Geometry: final body of the model. Coordinates: model frame, mm. A direction names the side the tool comes from. Give positions to 0.01 mm unless a question says otherwise; leave off trailing zeros. Write each loop counter-clockwise with the first axis right and the second up, starting at its lowest first coordinate (ties: lowest second). Pieces come first, ordered by that corner, then holes.
Q1. Cut plane D-D on z = 16. Return the cut outline in (x, y) (3 decimals).
Q2. Reachability of faces 4 (the face through (-20.003, 7.013, 17.546)), 5 (the face through (-19.284, -19.4, 15.944)), 6 (the face through (0, -12.5, 3)) from +Z, -Z, +X, -X, +Y, -Y: full face, straight path, thin tool, end or side. Return the list, or none.
Q3. Line query: L1, parallel to X at y = -1.5, z = 13 (3 decimals); L2, parallel to Y at x = 13, z = 3.25; L3, parallel to Y at x = 0, z = 8.95. Output: solid intervals per line, ascending.
Q4. Cut plane C-C on x = 10. Return the cut outline in (y, z) (3 decimals).
Q5. Cut plane B-B on z = 3. Return the cut outline in (x, y), plus the area to 3 significant figures.
Q6. Draft query along Y for faces 1 (the face through (0, 22.5, 10)), 2 (the face through (3, 0, 6)), 3 (the face through (-22.5, 0, 10)). Return one class per face: pulls with the +Y half, pulls with the -Y half, needs draft (parallel to the pull), parting line crosses it, or undercut.
Q7. Cut plane A-A on y = -7.5. Return the cut outline in (x, z) (3 decimals), plus the area to 3 significant figures.
Q8. Pin query (flat end, axial travel): pin 1 (1.8 mm diameter, centred on x = 12.5, y = -12.5, fed in from -Z); pin 2 (3.5 mm diameter, centred on x = -12.5, y = -12.5, fed in from +Z); pin 3 (1.9 mm diameter, centred on x = 0, y = 0, fed in from -Z); pin 4 (6.5 mm diameter, centred on x = -17.575, y = 17.575, fed in from -Z). Return the tip coordinate at first contact, or that it passes through.
Autodesk Inventor part; units mm, degrees
ref_plane "YZ Plane" through (0, 0, 0) normal (1, 0, 0) x (0, 1, 0)
ref_plane "XZ Plane" through (0, 0, 0) normal (0, 1, 0) x (-1, 0, 0)
ref_plane "XY Plane" through (0, 0, 0) normal (0, 0, 1) x (1, 0, 0)
sketch "Sketch1" plane through (0, 0, 0) normal (0, 0, 1) x (1, 0, 0)
  line L0 (0, 31.5) -> (0, -31.5) construction
  line L1 (-31.5, 0) -> (31.5, 0) construction
  line L2 (-22.5, 22.5) -> (22.5, 22.5)
  line L3 (22.5, 22.5) -> (22.5, -22.5)
  line L4 (22.5, -22.5) -> (-22.5, -22.5)
  line L5 (-22.5, -22.5) -> (-22.5, 22.5)
  point P0 (0, 0)
  dimension "d0" = 45
  dimension "d1" = 45
extrude "Extrusion1" add sketch "Sketch1" along normal blind 20
sketch "Sketch4" plane through (0, 0, 20) normal (0, 0, 1) x (1, 0, 0)
  line L0 (-31.5, 0) -> (31.5, 0) construction
  line L1 (0, 31.5) -> (0, -31.5) construction
  line L2 (-17.575, 17.575) -> (17.575, 17.575) construction
  line L3 (17.575, 17.575) -> (17.575, -17.575) construction
  line L4 (17.575, -17.575) -> (-17.575, -17.575) construction
  line L5 (-17.575, -17.575) -> (-17.575, 17.575) construction
  point P0 (0, 0)
  dimension "d15" = 35.15
  dimension "d16" = 35.15
hole "Hole2" at (-17.575, 17.575, 20) at (17.575, 17.575, 20) at (17.575, -17.575, 20) at (-17.575, -17.575, 20) at (-17.575, 17.575, 20) at (17.575, 17.575, 20) direction (0, 0, -1) diameter 5 depth 8
sketch "Sketch5" plane through (0, 0, 20) normal (0, 0, 1) x (1, 0, 0)
  circle A0 centre (-17.575, 17.575) radius 2.5
  circle A1 centre (17.575, -17.575) radius 2.5
  line L0 (-17.575, 17.575) -> (17.575, 17.575)
  line L1 (17.575, 17.575) -> (17.575, -17.575)
  line L2 (17.575, -17.575) -> (-17.575, -17.575)
  line L3 (-17.575, -17.575) -> (-17.575, 17.575)
  point P0 (0, 0)
extrude "Extrusion3" cut sketch "Sketch5" against normal blind 8 contours L0 L1 A1 L2 L3 A0 | A0 L3 L0 | L1 L2 A1 picked at (-15.9292, 17.3896) picked at (17.028, -16.0118)
sketch "Sketch6" plane through (-22.5, -22.5, 0) normal (-1, 0, 0) x (0, 0, 1)
  line L0 (0, 45) -> (20, 45)
  line L1 (0, 0) -> (20, 0)
  line L2 (20, 7.425) -> (12, 7.425) construction
  line L3 (20, 37.575) -> (20, 7.425) construction
  line L4 (12, 37.575) -> (20, 37.575) construction
  line L5 (12, 7.425) -> (12, 37.575) construction
  line L6 (16, 37.575) -> (16, 7.425) construction
  point P0 (0, 22.5)
  point P1 (16, 30)
  point P2 (16, 15)
  dimension "d26" = 15
  dimension "d27" = 15
hole "Hole3" at (-22.5, 7.5, 16) at (-22.5, -7.5, 16) direction (1, 0, 0) diameter 3.242 end up to surface
sketch "Sketch8" plane through (0, 0, 0) normal (0, 0, -1) x (-1, 0, 0)
  line L0 (22.5, 22.5) -> (-22.5, 22.5) construction
  line L1 (-22.5, 22.5) -> (-22.5, -22.5) construction
  line L2 (-22.5, -22.5) -> (22.5, -22.5) construction
  line L3 (22.5, -22.5) -> (22.5, 22.5) construction
  line L4 (0, -38.5) -> (0, 38.5) construction
  line L5 (-38.5, 0) -> (38.5, 0) construction
  line L6 (-12.5, -12.5) -> (12.5, -12.5)
  line L7 (12.5, -12.5) -> (12.5, 12.5)
  line L8 (12.5, 12.5) -> (-12.5, 12.5)
  line L9 (-12.5, 12.5) -> (-12.5, -12.5)
  point P0 (0, 0)
  dimension "d44" = 25
  dimension "d45" = 25
extrude "Extrusion4" cut sketch "Sketch8" against normal blind 6
sketch "Sketch9" plane through (0, 0, 0) normal (0, 0, -1) x (-1, 0, 0)
  line L0 (12.5, 12.5) -> (12.5, -12.5) construction
  line L1 (12.5, -12.5) -> (-12.5, -12.5) construction
  line L2 (-12.5, -12.5) -> (-12.5, 12.5) construction
  line L3 (-12.5, 12.5) -> (12.5, 12.5) construction
  line L4 (22.5, 22.5) -> (-22.5, 22.5) construction
  line L5 (-22.5, 22.5) -> (-22.5, -22.5) construction
  line L6 (-22.5, -22.5) -> (22.5, -22.5) construction
  line L7 (22.5, -22.5) -> (22.5, 22.5) construction
  line L8 (12.5, -12.5) -> (-12.5, -12.5) construction
  point P0 (0, 0)
hole "Hole5" at (-12.5, 12.5, 0) at (-12.5, -12.5, 0) at (12.5, -12.5, 0) at (12.5, 12.5, 0) direction (0, 0, 1) diameter 3 depth 6
sketch "Sketch10" plane through (0, 0, 6) normal (0, 0, -1) x (-1, 0, 0)
  point P0 (0, 0)
  point P1 (0, 0)
hole "Hole6" at (0, 0, 6) direction (0, 0, 1) diameter 3.242 depth 4 tip angle 118
properties part number "Large-cuvette-mount-40mm-V3" material "PC/ABS Plastic"
Data:
1. outline: (-22.5, -22.5) - (22.5, -22.5) - (22.5, 22.5) - (-22.5, 22.5) - (-22.5, 9.121) - (-17.575, 9.121) - (-17.575, 15.075) arc R2.5 cw (long way) to (-15.075, 17.575) - (15.075, 17.575) arc R2.5 cw (long way) to (17.575, 15.075) - (17.575, -15.075) arc R2.5 cw (long way) to (15.075, -17.575) - (-15.075, -17.575) arc R2.5 cw (long way) to (-17.575, -15.075) - (-17.575, -9.121) - (-22.5, -9.121) - close; (-22.5, -5.879) - (-17.575, -5.879) - (-17.575, 5.879) - (-22.5, 5.879) - close
2. face 4: -X
2. face 5: +Z
2. face 6: -Z
3. L1: x = -22.5 to -17.575, 17.575 to 22.5
3. L2: y = -22.5 to -13.91, -11.09 to 11.09, 13.91 to 22.5
3. L3: y = -22.5 to -1.62, 1.62 to 22.5
4. outline: (-22.5, 0) - (-12.5, 0) - (-12.5, 6) - (12.5, 6) - (12.5, 0) - (22.5, 0) - (22.5, 20) - (17.575, 20) - (17.575, 12) - (-17.575, 12) - (-17.575, 20) - (-22.5, 20) - close
5. outline: (-22.5, -22.5) - (22.5, -22.5) - (22.5, 22.5) - (-22.5, 22.5) - close; hole (-12.5, -11) arc R1.5 ccw (long way) to (-11, -12.5) - (11, -12.5) arc R1.5 ccw (long way) to (12.5, -11) - (12.5, 11) arc R1.5 ccw (long way) to (11, 12.5) - (-11, 12.5) arc R1.5 ccw (long way) to (-12.5, 11) - close
5. area: 1,380 mm2
6. face 1: pulls with the +Y half
6. face 2: undercut
6. face 3: needs draft
7. outline: (-22.5, 0) - (-12.5, 0) - (-12.5, 6) - (12.5, 6) - (12.5, 0) - (22.5, 0) - (22.5, 20) - (17.575, 20) - (17.575, 12) - (-17.575, 12) - (-17.575, 14.379) - (-22.5, 14.379) - close; (-22.5, 17.621) - (-17.575, 17.621) - (-17.575, 20) - (-22.5, 20) - close
7. area: 453 mm2
8. pin 1: stops at z = 6
8. pin 2: stops at z = 12
8. pin 3: stops at z = 10.4
8. pin 4: stops at z = 0
